```python
from build123d import *

# Parameters (mm, degrees)
F0_W     = 76.2
F0_H     = 50.8
F1_DEPTH = 25.4
F2_R     = 3.302
F3_DEPTH = 19.05
F4_R     = 5.08


with BuildPart() as f1:
    # F0 (on Front) → F1 (new body)
    with BuildSketch(Plane.XZ):
        with Locations((38.1, 25.4)):
            Rectangle(F0_W, F0_H)
    extrude(amount=F1_DEPTH)

    # F2 (on face) → F3 (cut)
    with BuildSketch(Plane.XZ.offset(25.4)):
        with Locations((69.85, 6.35)):
            Circle(F2_R)
        with Locations((69.85, 25.4)):
            Circle(F2_R)
        with Locations((69.85, 44.45)):
            Circle(F2_R)
        with Locations((48.683333, 6.35)):
            Circle(F2_R)
        with Locations((48.683333, 25.4)):
            Circle(F2_R)
        with Locations((48.683333, 44.45)):
            Circle(F2_R)
        with Locations((27.516667, 6.35)):
            Circle(F2_R)
        with Locations((27.516667, 25.4)):
            Circle(F2_R)
        with Locations((27.516667, 44.45)):
            Circle(F2_R)
        with Locations((6.35, 6.35)):
            Circle(F2_R)
        with Locations((6.35, 25.4)):
            Circle(F2_R)
        with Locations((6.35, 44.45)):
            Circle(F2_R)
    extrude(amount=-F3_DEPTH, mode=Mode.SUBTRACT)

    # F4
    f4_edges = [f1.edges().sort_by_distance(p)[0] for p in [
        (76.2, -12.7, 50.8),
        (0, -12.7, 50.8),
        (0, -12.7, 0),
        (76.2, -12.7, 0),
    ]]
    fillet(f4_edges, radius=F4_R)


solid = f1.part
```
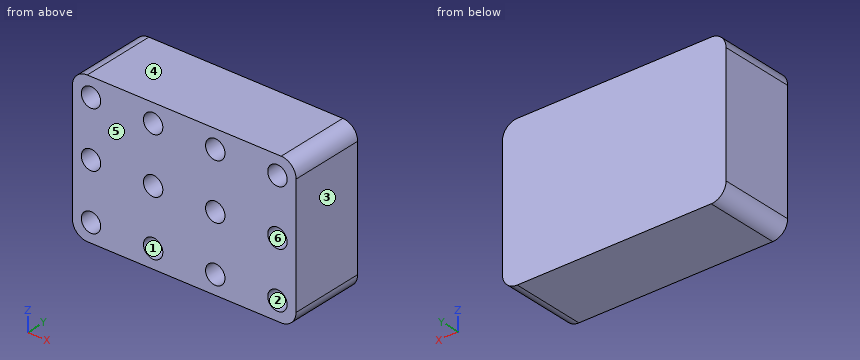
Read the model definition and answer for the solid it produces. Units are mm, in the model's axes. Face numbers are marked on the shaded views. A direction names the side the tool comes from. Give positions to 0.01 mm unless a question says otherwise; leave off trailing zeros. Loops run counter-clockwise (first coordinate to the right, second up) from the corner with the lowest first, then second, coordinate; pieces in that order, holes last.
Item 1: For the marked faces 5 and 6, determine the directions among +Z, -Z, +X, -X, +Y, -Y from which every point of the face is accessible in a straight line to the end or side of a thin tool.
Item 2: Each of these flat-tipped pins is pushed along its axis until it touches: pin 1 Ø3.5 at (x, z) = (27.5, 7.5) entering from -Y; pin 2 Ø8.5 at (x, z) = (6.35, 25.4) entering from -Y. Where does it stop, or does it pass through?
Item 3: The mould has two halves that part along Z. Classify the marked faces 1, 2, 3 and 4: released by +Z, released by -Z, zero draft, split by the parting line, or undercut.
Item 4: Find the intervals of material crossed by line 1 along Z through (x, y) = (69.85, -12.5); line 2 along Z through (x, y) = (26, -14); line 3 along X through (y, z) = (-6.75, 46.5), in increasing order.
Item 5: The part is cut by section B-B (x = 6.35). Write down the section's boundary in (y, z).
Item 6: The part is cut by section C-C (z = 7.5). Write down the section's boundary in (x, y).
Item 7: The part is cut by section D-D (x = 27). Write down the section's boundary in (y, z).
Item 8: The part is cut by section A-A (z = 25.4). Write down the section's boundary in (x, y), and give its area (3 significant figures).
Taken from the geometry:
1. face 5: +Z, -Z, +X, -X, -Y
1. face 6: -Y
2. pin 1: stops at y = -6.35
2. pin 2: stops at y = -25.4
3. face 1: undercut
3. face 2: undercut
3. face 3: zero draft
3. face 4: released by +Z
4. line 1: z = 0 to 3.05, 9.65 to 22.1, 28.7 to 41.15, 47.75 to 50.8
4. line 2: z = 0 to 3.42, 9.28 to 22.47, 28.33 to 41.52, 47.38 to 50.8
4. line 3: x = 0.06 to 3.76, 8.94 to 24.93, 30.11 to 46.09, 51.27 to 67.26, 72.44 to 76.14
5. outline: (-25.4, 0) - (0, 0) - (0, 50.8) - (-25.4, 50.8) - (-25.4, 47.75) - (-6.35, 47.75) - (-6.35, 41.15) - (-25.4, 41.15) - (-25.4, 28.7) - (-6.35, 28.7) - (-6.35, 22.1) - (-25.4, 22.1) - (-25.4, 9.65) - (-6.35, 9.65) - (-6.35, 3.05) - (-25.4, 3.05) - close
6. outline: (0, -25.4) - (3.25, -25.4) - (3.25, -6.35) - (9.45, -6.35) - (9.45, -25.4) - (24.42, -25.4) - (24.42, -6.35) - (30.61, -6.35) - (30.61, -25.4) - (45.59, -25.4) - (45.59, -6.35) - (51.78, -6.35) - (51.78, -25.4) - (66.75, -25.4) - (66.75, -6.35) - (72.95, -6.35) - (72.95, -25.4) - (76.2, -25.4) - (76.2, 0) - (0, 0) - close
7. outline: (-25.4, 0) - (0, 0) - (0, 50.8) - (-25.4, 50.8) - (-25.4, 47.71) - (-6.35, 47.71) - (-6.35, 41.19) - (-25.4, 41.19) - (-25.4, 28.66) - (-6.35, 28.66) - (-6.35, 22.14) - (-25.4, 22.14) - (-25.4, 9.61) - (-6.35, 9.61) - (-6.35, 3.09) - (-25.4, 3.09) - close
8. outline: (0, -25.4) - (3.05, -25.4) - (3.05, -6.35) - (9.65, -6.35) - (9.65, -25.4) - (24.21, -25.4) - (24.21, -6.35) - (30.82, -6.35) - (30.82, -25.4) - (45.38, -25.4) - (45.38, -6.35) - (51.99, -6.35) - (51.99, -25.4) - (66.55, -25.4) - (66.55, -6.35) - (73.15, -6.35) - (73.15, -25.4) - (76.2, -25.4) - (76.2, 0) - (0, 0) - close
8. area: 1,430 mm2
